Can you work these out from the model? Positions are in its coordinate system, mm. A direction names the side the tool comes from. Give positions to 0.01 mm unless a question says otherwise; leave off trailing zeros. Loops run counter-clockwise (first coordinate to the right, second up) from the corner with the lowest first, then second, coordinate; pieces in that order, holes last. Notation, with made-up numbers: (-39, 1) - (18, 1) arc R14 cw to (18, 13) - close; hole circle Ø9 at (34.25, 47.25). An arc over 180 degrees is marked (long way). Answer in a Markdown table with one row per item.
from build123d import *

# Parameters (mm, degrees)
ESQUISSE1_W             = 20
ESQUISSE1_H             = 20
BOSS_EXTRU_1_DEPTH      = 35
COQUE2_T                = -2
CONG_1_R                = 0.5
ESQUISSE2_R             = 6
BOSS_EXTRU_2_DEPTH      = 33
ESQUISSE3_R             = 5
ENL_V_MAT_EXTRU_3_DEPTH = 33
CONG_2_R                = 0.8


with BuildPart() as part:
    # Esquisse1 → Boss.-Extru.1 (new body)
    with BuildSketch(Plane.XY):
        Rectangle(ESQUISSE1_W, ESQUISSE1_H)
    extrude(amount=BOSS_EXTRU_1_DEPTH)

    # Coque2
    coque2_openings = [part.faces().sort_by_distance(p)[0] for p in [
        (0, 0, 35),
    ]]
    offset(amount=COQUE2_T, openings=coque2_openings, kind=Kind.INTERSECTION)

    # Congé1
    cong_1_edges = [part.edges().sort_by_distance(p)[0] for p in [
        (-8, 8, 18.5),
        (-8, -8, 18.5),
        (8, -8, 18.5),
        (8, 8, 18.5),
        (-10, 10, 17.5),
        (10, 10, 17.5),
        (10, -10, 17.5),
        (-10, -10, 17.5),
    ]]
    fillet(cong_1_edges, radius=CONG_1_R)

    # Esquisse2 → Boss.-Extru.2 (add)
    with BuildSketch(Plane.XY.offset(2)):
        with Locations(Location((0, 0, 0), (0, 0, 180))):
            Circle(ESQUISSE2_R)
    extrude(amount=BOSS_EXTRU_2_DEPTH)

    # Esquisse3 → Enlèv. mat.-Extru.3 (cut)
    with BuildSketch(Plane.XY.offset(35)):
        Circle(ESQUISSE3_R)
    extrude(amount=-ENL_V_MAT_EXTRU_3_DEPTH, mode=Mode.SUBTRACT)

    # Congé2
    cong_2_edges = [part.edges().sort_by_distance(p)[0] for p in [
        (6, 0, 2),
    ]]
    fillet(cong_2_edges, radius=CONG_2_R)


solid = part.part
Q1. Imagine slicing it at B-B, the plane x = 0. Write out the boundary of the cut face in (y, z), and give its area (3 significant figures).
Checked values:
| item | result |
|---|---|
| outline | (-10, 0) - (10, 0) - (10, 35) - (8, 35) - (8, 2) - (6.8, 2) arc R0.8 cw to (6, 2.8) - (6, 35) - (5, 35) - (5, 2) - (-5, 2) - (-5, 35) - (-6, 35) - (-6, 2.8) arc R0.8 cw to (-6.8, 2) - (-8, 2) - (-8, 35) - (-10, 35) - close |
| area | 238 mm² |
Q2. If I drill on line 1 (Y direction, x = 0, z = 15.5); line 2 (X direction, y = 0.25, z = 4); line 3 (Y direction, x = 5.25, z = 29), over which ranges is the centre line in solid material (lowest first)? Write a range as [from, to].
Checked values:
| item | result |
|---|---|
| line 1 | y = [-10, -8], [-6, -5], [5, 6], [8, 10] |
| line 2 | x = [-10, -8], [-5.99, -4.99], [4.99, 5.99], [8, 10] |
| line 3 | y = [-10, -8], [-2.9, 2.9], [8, 10] |
Q3. Imagine slicing it at A-A, the plane z = 26.5. Write out the boundary of the cut face in (x, y).
Checked values:
| item | result |
|---|---|
| outline | (-10, -9.5) arc R0.5 ccw to (-9.5, -10) - (9.5, -10) arc R0.5 ccw to (10, -9.5) - (10, 9.5) arc R0.5 ccw to (9.5, 10) - (-9.5, 10) arc R0.5 ccw to (-10, 9.5) - close; circle Ø12 at (0, 0); hole (-8, -7.5) arc R0.5 ccw to (-7.5, -8) - (7.5, -8) arc R0.5 ccw to (8, -7.5) - (8, 7.5) arc R0.5 ccw to (7.5, 8) - (-7.5, 8) arc R0.5 ccw to (-8, 7.5) - close; hole circle Ø10 at (0, 0) |
Q4. For pin 1 (4 mm diameter, centred on x = -1.5, y = 2, fed in from +Z), with a flat end and sliding along its axis, tell me the tip position at first contact or that it passes through.
Checked values:
| item | result |
|---|---|
| pin 1 | stops at z = 2 |
Q5. On a 3-axis mill with a long thin cutter (end or side, diameter ignored), from which of +Z, -Z, +X, -X, +Y, -Y can I reach the whole of each face in a straight line? I mean faces 5 (the face through (-1.08, -4.88, 18.73)), 6 (the face through (0, -10, 17)). Say none if no direction works.
Checked values:
| item | result |
|---|---|
| face 5 | +Z |
| face 6 | +Z, -Z, +X, -X, -Y |
Q6. If we mould it in two halves opening along X, with no side actions, what happens to faces 1 (the face through (0, 10, 17)), 2 (the face through (-8, 0, 18)), 3 (the face through (0, 8, 18)), 4 (the face through (-10, 0, 17))? For each: released by +X, released by -X, zero draft, split by the parting line, or undercut.
Checked values:
| item | result |
|---|---|
| face 1 | zero draft |
| face 2 | undercut |
| face 3 | undercut |
| face 4 | released by -X |
